```python
from build123d import *

# Parameters (mm, degrees)
IZIM1_R                                           = 44
IZIM1_R_2                                         = 22.5
Y_KSEKLIK_EKSTR_ZYON1_DEPTH                       = 12
M8_ALT_GEN_ALYAN_BA_L_K_R_VIDA_IN_HAV_D           = 9
M8_ALT_GEN_ALYAN_BA_L_K_R_VIDA_IN_HAV_DEPTH       = 22.25
M8_ALT_GEN_ALYAN_BA_L_K_R_VIDA_IN_HAV_CBORE_D     = 15
M8_ALT_GEN_ALYAN_BA_L_K_R_VIDA_IN_HAV_CBORE_DEPTH = 8.6
M8_ALT_GEN_ALYAN_BA_L_K_R_VIDA_IN_HAV_TIP         = 2.703872786


with BuildPart() as part:
    # Çizim1 → Yükseklik-Ekstrüzyon1 (new body)
    with BuildSketch(Plane.XY):
        Circle(IZIM1_R)
        Circle(IZIM1_R_2, mode=Mode.SUBTRACT)
    extrude(amount=Y_KSEKLIK_EKSTR_ZYON1_DEPTH)

    # M8 Altıgen Alyan Başlı Kör Vida İçin Havşa1
    with Locations(Plane.XY.offset(12)):
        with Locations((0, -35), (-35, 0), (0, 35), (35, 0)):
            CounterBoreHole(M8_ALT_GEN_ALYAN_BA_L_K_R_VIDA_IN_HAV_D / 2, M8_ALT_GEN_ALYAN_BA_L_K_R_VIDA_IN_HAV_CBORE_D / 2, M8_ALT_GEN_ALYAN_BA_L_K_R_VIDA_IN_HAV_CBORE_DEPTH, depth=M8_ALT_GEN_ALYAN_BA_L_K_R_VIDA_IN_HAV_DEPTH)
            with Locations((0, 0, -(M8_ALT_GEN_ALYAN_BA_L_K_R_VIDA_IN_HAV_DEPTH + M8_ALT_GEN_ALYAN_BA_L_K_R_VIDA_IN_HAV_TIP / 2))):  # 118° drill point
                Cone(0, M8_ALT_GEN_ALYAN_BA_L_K_R_VIDA_IN_HAV_D / 2, M8_ALT_GEN_ALYAN_BA_L_K_R_VIDA_IN_HAV_TIP, mode=Mode.SUBTRACT)


solid = part.part
```
For this review, take the finished solid that the model builds, in its own axes (mm). A direction names the side the tool comes from. Round coordinates to 2 decimals unless told otherwise and drop trailing zeros. Write each loop counter-clockwise with the first axis right and the second up, starting at its lowest first coordinate (ties: lowest second). Pieces come first, ordered by that corner, then holes.
1) Mouldability with a two-part tool opening along X and no side actions: class faces 1 (the face through (-9.538, -42.954, 5.916)), 2 (the face through (27.507, 0.33, 7.76)), 3 (the face through (-20.2, 10.4, 0)) as +X half, -X half, draft (parallel to the pull), parting line (faces both ways), or undercut.
Answer below:
face 1: parting line
face 2: undercut
face 3: draft
2) Take a section at C-C on z = 2.25. Give the boundary of the cut face in (x, y), then the cut area to 3 significant figures.
Answer below:
outline: circle Ø88 at (0, 0); hole circle Ø9 at (-35, 0); hole circle Ø45 at (0, 0); hole circle Ø9 at (0, -35); hole circle Ø9 at (0, 35); hole circle Ø9 at (35, 0)
area: 4,240 mm2
3) Take a section at A-A on x = 0. Give the boundary of the cut face in (y, z).
Answer below:
outline: (-44, 0) - (-39.5, 0) - (-39.5, 3.4) - (-42.5, 3.4) - (-42.5, 12) - (-44, 12) - close; (-30.5, 0) - (-22.5, 0) - (-22.5, 12) - (-27.5, 12) - (-27.5, 3.4) - (-30.5, 3.4) - close; (22.5, 0) - (30.5, 0) - (30.5, 3.4) - (27.5, 3.4) - (27.5, 12) - (22.5, 12) - close; (39.5, 0) - (44, 0) - (44, 12) - (42.5, 12) - (42.5, 3.4) - (39.5, 3.4) - close
4) Take a section at D-D on x = -16.5. Give the boundary of the cut face in (y, z), then the cut area to 3 significant figures.
Answer below:
outline: (-40.79, 0) - (-15.3, 0) - (-15.3, 12) - (-40.79, 12) - close; (15.3, 0) - (40.79, 0) - (40.79, 12) - (15.3, 12) - close
area: 612 mm2
5) Insertion check: pin 1 Ø13.5 at (x, y) = (0, -35) entering from -Z; pin 2 Ø1.5 at (y, z) = (-13, 3) entering from -X; pin 3 Ø4.5 at (x, y) = (-38.5, -2) entering from +Z; pin 4 Ø1.5 at (y, z) = (-9.5, 10) entering from +X. Each pin has a flat end and moves straight along its axis. Give the tip position at first contact, or say it passes through.
Answer below:
pin 1: stops at z = 0
pin 2: stops at x = -42.26
pin 3: stops at z = 3.4
pin 4: stops at x = 43.12
6) Machinability: for faces 4 (the face through (0.98, 30.61, 1.68)), 5 (the face through (5, -35, 3.4)), which of the approach directions +Z, -Z, +X, -X, +Y, -Y give a long, thin tool a straight path to every point of the face, cutting with its end or side? Answer none if there is none.
Answer below:
face 4: +Z, -Z
face 5: +Z
7) For line 1 along Y through (x, z) = (0, 1.75); line 2 along Y through (x, z) = (2.5, 6); line 3 along Z through (x, y) = (5, -34), list the stretches that pass through material, from the lowest coordinate up.
Answer below:
line 1: y = -44 to -39.5, -30.5 to -22.5, 22.5 to 30.5, 39.5 to 44
line 2: y = -43.93 to -42.07, -27.93 to -22.36, 22.36 to 27.93, 42.07 to 43.93
line 3: z = 0 to 3.4
